Can you work these out from the drawing? Everything is in mm from the part's minimum corner. A direction names the side the tool comes from. Round coordinates to 2 decimals unless told otherwise and drop trailing zeros. Loops run counter-clockwise (first coordinate to the right, second up) from the corner with the lowest first, then second, coordinate; pieces in that order, holes last. Notation, with made-up numbers: (60, 40.5) -> (106, 40.5) arc R29 ccw to (106, 72.5) -> close; hole circle Ø1 at (-16, -7.5). An arc over 180 degrees is marked (long way). One line per item, written item: value.
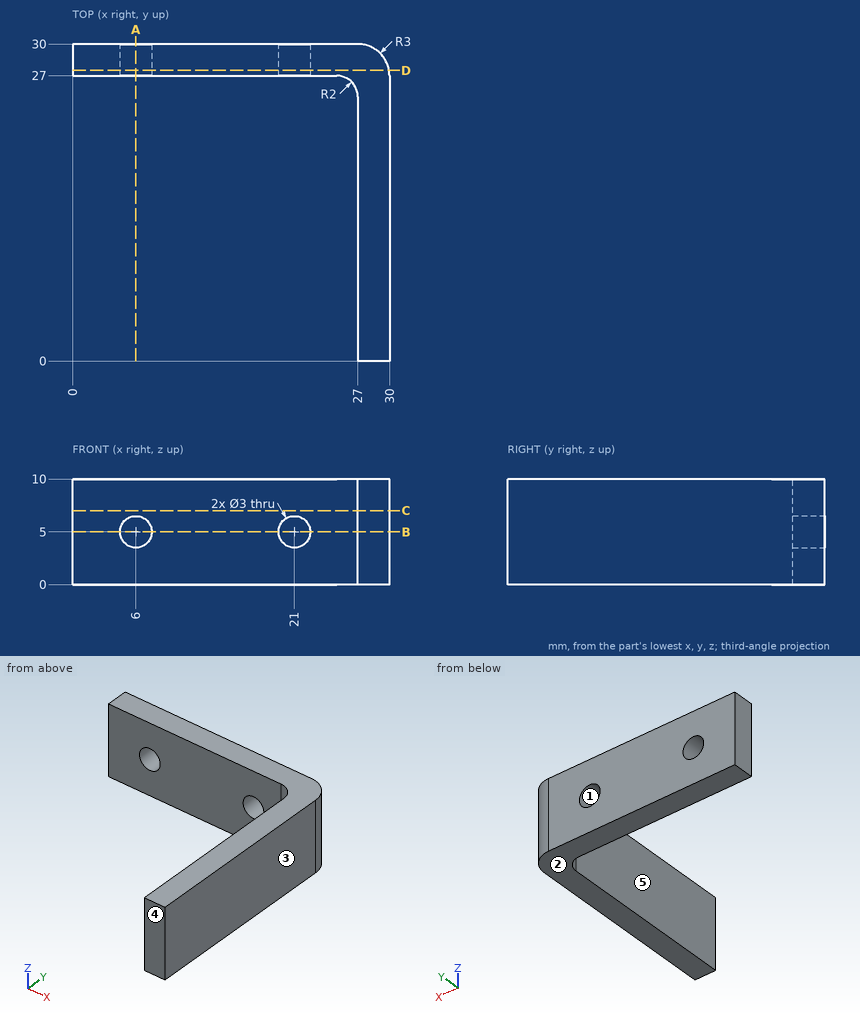
Item 1: For the marked faces 4 and 5, which set-ups out of +Z, -Z, +X, -X, +Y, -Y let a thin tool reach every point of the face, with its end or its side?
Output:
face 4: +Z, -Z, +X, -X, -Y
face 5: +Z, -Z, -X, -Y
Item 2: If we section it at A-A on x = 6: List the corners of the cut face in (y, z) for me, plus the area to 3 significant figures.
Output:
outline: (27, 0) -> (30, 0) -> (30, 3.5) -> (27, 3.5) -> close; (27, 6.5) -> (30, 6.5) -> (30, 10) -> (27, 10) -> close
area: 21.0 mm²
Item 3: If we section it at C-C on z = 7: List the corners of the cut face in (x, y) for me.
Output:
outline: (0, 27) -> (25, 27) arc R2 cw to (27, 25) -> (27, 0) -> (30, 0) -> (30, 27) arc R3 ccw to (27, 30) -> (0, 30) -> close
Item 4: If we section it at B-B on z = 5: List the corners of the cut face in (x, y) for me.
Output:
outline: (0, 27) -> (4.5, 27) -> (4.5, 30) -> (0, 30) -> close; (7.5, 27) -> (19.5, 27) -> (19.5, 30) -> (7.5, 30) -> close; (22.5, 27) -> (25, 27) arc R2 cw to (27, 25) -> (27, 0) -> (30, 0) -> (30, 27) arc R3 ccw to (27, 30) -> (22.5, 30) -> close
Item 5: If we section it at D-D on y = 27.5: List the corners of the cut face in (x, z) for me, plus the area to 3 significant figures.
Output:
outline: (0, 0) -> (29.96, 0) -> (29.96, 10) -> (0, 10) -> close; hole circle Ø3 at (6, 5); hole circle Ø3 at (21, 5)
area: 285 mm²
Item 6: Will these pins go through, and if not, where does the flat tip stop? pin 1 Ø5 at (y, z) = (7.5, 6.5) entering from -X; pin 2 Ø4 at (x, z) = (23.5, 7.5) entering from -Y; pin 3 Ø1 at (x, z) = (23.5, 2) entering from -Y.
Output:
pin 1: stops at x = 27
pin 2: stops at y = 26.94
pin 3: stops at y = 27
Item 7: If we mould it in two halves opening along X, with no side actions, what happens to the marked faces 1, 2 and 3? For each: released by +X, released by -X, zero draft, split by the parting line, or undercut.
Output:
face 1: undercut
face 2: zero draft
face 3: released by +X
Item 8: I need wall thicknesses on line 1 (Z direction, x = 6, y = 28.8); line 2 (X direction, y = 28.3, z = 5); line 3 (X direction, y = 28, z = 5). Which ranges of each line are inside material? Lowest first, please. Write a range as from..to.
Output:
line 1: z = 0..3.5, 6.5..10
line 2: x = 0..4.5, 7.5..19.5, 22.5..29.7
line 3: x = 0..4.5, 7.5..19.5, 22.5..29.83
